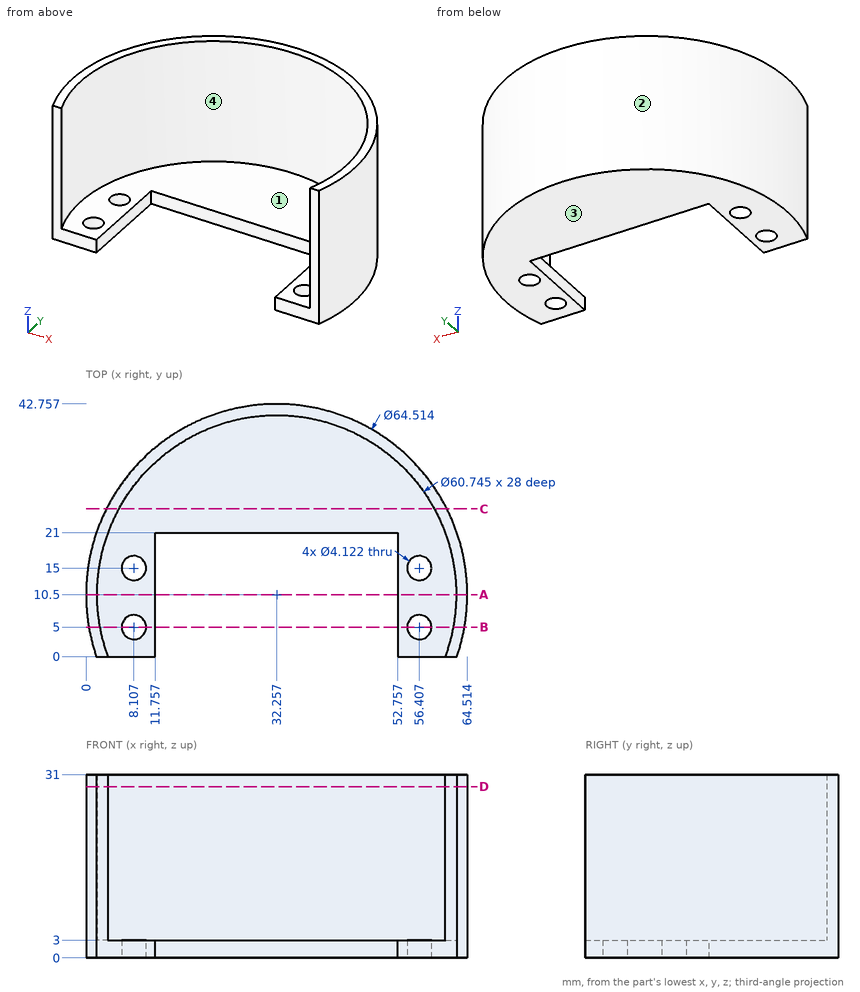
For this review, use the dimensioned drawing (mm, ordinates from the lowest corner) and the shaded views. Coordinates: 2 decimals unless noted, no trailing zeros. Write each loop counter-clockwise with the first axis right and the second up, starting at its lowest first coordinate (ties: lowest second). Pieces come first, ordered by that corner, then holes. Notation, with made-up numbers: (49.5, 14.5) - (69.5, 14.5) arc R25 cw to (69.5, 45.5) - close; hole circle Ø3 at (48, 43). An arc over 180 degrees is marked (long way). Answer in a Markdown table with one row per item. Add a question column.
Q1. Clearance check with flat-ended pins moving along their axes: pin 1 (3.5 mm diameter, centred on y = 5.5, z = 1.5, fed in from -X); pin 2 (3.5 mm diameter, centred on x = 56.41, y = 15, fed in from +Z); pin 3 (6 mm diameter, centred on x = 8, z = 25, fed in from +Y); pin 4 (20.5 mm diameter, centred on x = 34.5, y = 20, fed in from +Z). State where each tip first meets the part, or that it passes through.
Q2. Consider section D-D on z = 29. Give the boundary of the cut face in (x, y) (1 decimal).
Q3. Consider section A-A on y = 10.5. Give the boundary of the cut face in (x, z).
Q4. Consider section C-C on y = 25. Give the boundary of the cut face in (x, z) (1 decimal), then the cut area to 3 significant figures.
Q5. Consider section B-B on y = 5. Give the boundary of the cut face in (x, z) (1 decimal).
Q6. To check wall thickness, follow line 1 along X through (y, z) = (10, 19) (1 decimal); line 2 along X through (y, z) = (24.5, 13.5) (1 decimal); line 3 along Z through (x, y) = (11, 25). State the ranges of each line that lie inside material, in increasing order. Write a range as from..to.
Q7. Draft analysis for pull direction X (two halves, no side actions). For the marked faces 1, 2, 3 and 4, state which applies: +X half, -X half, draft (parallel to the pull), parting line (faces both ways), or undercut.
Answers below:
| question | item | result |
|---|---|---|
| 1 | pin 1 | x = 0.16 |
| 1 | pin 2 | through |
| 1 | pin 3 | y = 34.76 |
| 1 | pin 4 | z = 3 |
| 2 | outline | (1.8, 0) - (3.8, 0) arc R30.4 cw (long way) to (60.8, 0) - (62.8, 0) arc R32.3 ccw (long way) to start |
| 3 | outline | (0, 0) - (11.76, 0) - (11.76, 3) - (1.88, 3) - (1.88, 31) - (0, 31) - close; (52.76, 0) - (64.51, 0) - (64.51, 31) - (62.63, 31) - (62.63, 3) - (52.76, 3) - close |
| 4 | outline | (3.4, 0) - (61.1, 0) - (61.1, 31) - (58.9, 31) - (58.9, 3) - (5.6, 3) - (5.6, 31) - (3.4, 31) - close |
| 4 | area | 292 mm² |
| 5 | outline | (0.5, 0) - (6, 0) - (6, 3) - (2.4, 3) - (2.4, 31) - (0.5, 31) - close; (10.2, 0) - (11.8, 0) - (11.8, 3) - (10.2, 3) - close; (52.8, 0) - (54.3, 0) - (54.3, 3) - (52.8, 3) - close; (58.5, 0) - (64, 0) - (64, 31) - (62.1, 31) - (62.1, 3) - (58.5, 3) - close |
| 6 | line 1 | 0..1.9, 62.6..64.5 |
| 6 | line 2 | 3.2..5.3, 59.2..61.3 |
| 6 | line 3 | 0..3 |
| 7 | face 1 | undercut |
| 7 | face 2 | parting line |
| 7 | face 3 | draft |
| 7 | face 4 | undercut |
